```python
from build123d import *

# Parameters (mm, degrees)
ENL_V_MAT_EXTRU_1_REACH             = 17.684
ESQUISSE2_W                         = 2
ESQUISSE2_H                         = 8
ENL_V_MAT_EXTRU_1_DIRECTION_2_REACH = 17.684


with BuildPart() as part:
    # Esquisse1 → Révolution1 (revolve)
    with BuildSketch(Plane.XY, mode=Mode.PRIVATE) as r_volution1_sk:
        with BuildLine():
            Line((0, 0), (-5, 0))
            Line((-5, 0), (-5, 4))
            Line((-5, 4), (-4.75, 4))
            Line((-4.75, 4), (-4.75, 14))
            Line((-4.75, 14), (-4.55, 14))
            Line((-4.55, 14), (-3, 10))
            Line((-3, 10), (-3, 6))
            ThreePointArc((-3, 6), (-2.121320344, 3.878679656), (0, 3))
            Line((0, 3), (0, 0))
        make_face()
    revolve(r_volution1_sk.sketch.rotate(Axis((0, -3.503417728, 0), (0, 1, 0)), 270), axis=Axis((0, -3.503417728, 0), (0, 1, 0)))

    # Esquisse2 → Enlèv. mat.-Extru.1 (cut, up to next)
    with BuildSketch(Plane(origin=(0, 0, 0), x_dir=(0, 0, -1), z_dir=(1, 0, 0)), mode=Mode.PRIVATE) as enl_v_mat_extru_1_sk1:
        with Locations((0, 10)):
            Rectangle(ESQUISSE2_W, ESQUISSE2_H)
    enl_v_mat_extru_1_tool1 = extrude(enl_v_mat_extru_1_sk1.sketch, amount=-ENL_V_MAT_EXTRU_1_REACH, mode=Mode.PRIVATE) & part.part
    add(enl_v_mat_extru_1_tool1.solids().sort_by_distance((0, 10, 0))[0], mode=Mode.SUBTRACT)

    # Esquisse2 → Enlèv. mat.-Extru.1 direction 2 (cut, up to next)
    with BuildSketch(Plane(origin=(0, 0, 0), x_dir=(0, 0, -1), z_dir=(1, 0, 0)), mode=Mode.PRIVATE) as enl_v_mat_extru_1_direction_2_sk1:
        with Locations((0, 10)):
            Rectangle(ESQUISSE2_W, ESQUISSE2_H)
    enl_v_mat_extru_1_direction_2_tool1 = extrude(enl_v_mat_extru_1_direction_2_sk1.sketch, amount=ENL_V_MAT_EXTRU_1_DIRECTION_2_REACH, mode=Mode.PRIVATE) & part.part
    add(enl_v_mat_extru_1_direction_2_tool1.solids().sort_by_distance((0, 10, 0))[0], mode=Mode.SUBTRACT)


solid = part.part
```
Here's how the part is built. I have some questions about the finished solid (model axes, mm). A direction names the side the tool comes from. Give positions to 0.01 mm unless a question says otherwise; leave off trailing zeros. Loops run counter-clockwise (first coordinate to the right, second up) from the corner with the lowest first, then second, coordinate; pieces in that order, holes last. Notation, with made-up numbers: (37, 2) -> (81, 2) arc R36 ccw to (81, 40) -> close; hole circle Ø3 at (63, -26.75). An arc over 180 degrees is marked (long way). Use one line per item in the form item = value. Start each with the question number.
1) Imagine slicing it at B-B (z = 0). Please give me the cut outline in (x, y), then the cut area to 3 significant figures.
2) Thinking about a two-plate mould opening in X: for faces 1 (the face through (4.88, 2.03, 1.08)), 2 (the face through (0, 8, -3)), 3 (the face through (4, 9, -1)), which applies, +X half, -X half, draft (parallel to the pull), parting line (faces both ways), or undercut?
3) Please list where these lines run through material, in increasing order: line 1 along Y through (x, z) = (3, -0.75); line 2 along X through (y, z) = (2.5, -4); line 3 along Z through (x, y) = (2.25, 11.75).
4) Imagine slicing it at A-A (y = 9.5). Please give me the cut outline in (x, z), then the cut area to 3 significant figures.
5) Imagine slicing it at D-D (y = 1.75). Please give me the cut outline in (x, z), then the cut area to 3 significant figures.
6) Which directions (+Z, -Z, +X, -X, +Y, -Y) give clear straight access to the entire face, cutting with the end or side of a thin tool? Please do faces 4 (the face through (0.068, 11.528, -3.591)), 5 (the face through (-4, 6, 0)), 6 (the face through (0, 0, 0)).
7) Imagine slicing it at C-C (x = 0). Please give me the cut outline in (y, z).
8) For P1, Ø2, axis at x = 4, y = 10, coming from the +Z side; P2, Ø6, axis at x = -2, y = 9.5, coming from the -Z side; P3, Ø3, axis at y = 12, z = -3.5, coming from the +X side, each with a flat end and sliding along its axis, tell me the tip position at first contact or that it passes through.
Check values:
q1.outline = (-5, 0) -> (5, 0) -> (5, 4) -> (4.75, 4) -> (4.75, 6) -> (3, 6) arc R3 cw to (-3, 6) -> (-4.75, 6) -> (-4.75, 4) -> (-5, 4) -> close
q1.area = 44.9 mm^2
q2.face_1 = parting line
q2.face_2 = undercut
q2.face_3 = draft
q3.line_1 = 0 to 6
q3.line_2 = -3 to 3
q3.line_3 = -4.18 to -2.91, 2.91 to 4.18
q4.outline = (-4.64, -1) arc R4.75 ccw to (4.64, -1) -> (2.83, -1) arc R3 cw to (-2.83, -1) -> close; (-4.64, 1) -> (-2.83, 1) arc R3 cw to (2.83, 1) -> (4.64, 1) arc R4.75 ccw to start
q4.area = 35.5 mm^2
q5.outline = circle Ø10 at (0, 0)
q5.area = 78.5 mm^2
q6.face_4 = +Y
q6.face_5 = +X, -X, +Y
q6.face_6 = +Z, -Z, +X, -X, -Y
q7.outline = (0, -5) -> (4, -5) -> (4, -4.75) -> (14, -4.75) -> (14, -4.55) -> (10, -3) -> (6, -3) arc R3 cw to (6, 3) -> (10, 3) -> (14, 4.55) -> (14, 4.75) -> (4, 4.75) -> (4, 5) -> (0, 5) -> close
q8.P1 = 3.68
q8.P2 = -4.75
q8.P3 = 4.31
